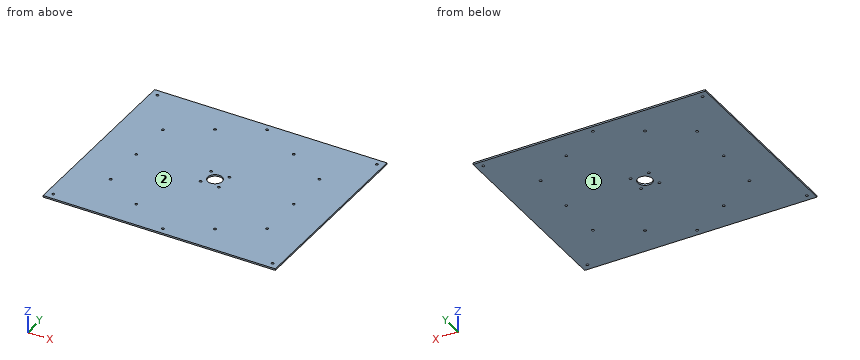
from build123d import *

# Parameters (mm, degrees)
F0_W     = 457.2
F0_H     = 381
F0_R     = 2.4892
F0_R_2   = 14.2875
F1_DEPTH = 3.175
F2_R     = 2.4892
F3_DEPTH = 3.176


with BuildPart() as f1:
    # F0 (on Top) → F1 (new body)
    with BuildSketch(Plane.XY):
        with Locations((228.6, 190.5)):
            Rectangle(F0_W, F0_H)
        with Locations((151.088372, 56.245922)):
            Circle(F0_R, mode=Mode.SUBTRACT)
        with Locations((74.620683, 101.6)):
            Circle(F0_R, mode=Mode.SUBTRACT)
        with Locations((210.639488, 172.539488)):
            Circle(F0_R, mode=Mode.SUBTRACT)
        with Locations((228.6, 12.7)):
            Circle(F0_R, mode=Mode.SUBTRACT)
        with Locations((306.111628, 56.245922)):
            Circle(F0_R, mode=Mode.SUBTRACT)
        with Locations((246.560512, 172.539488)):
            Circle(F0_R, mode=Mode.SUBTRACT)
        with Locations((382.579317, 101.6)):
            Circle(F0_R, mode=Mode.SUBTRACT)
        with Locations((73.576744, 190.5)):
            Circle(F0_R, mode=Mode.SUBTRACT)
        with Locations((74.620683, 279.4)):
            Circle(F0_R, mode=Mode.SUBTRACT)
        with Locations((210.639488, 208.460512)):
            Circle(F0_R, mode=Mode.SUBTRACT)
        with Locations((151.088372, 324.754078)):
            Circle(F0_R, mode=Mode.SUBTRACT)
        with Locations((228.6, 190.5)):
            Circle(F0_R_2, mode=Mode.SUBTRACT)
        with Locations((246.560512, 208.460512)):
            Circle(F0_R, mode=Mode.SUBTRACT)
        with Locations((383.623256, 190.5)):
            Circle(F0_R, mode=Mode.SUBTRACT)
        with Locations((382.579317, 279.4)):
            Circle(F0_R, mode=Mode.SUBTRACT)
        with Locations((306.111628, 324.754078)):
            Circle(F0_R, mode=Mode.SUBTRACT)
        with Locations((228.6, 368.3)):
            Circle(F0_R, mode=Mode.SUBTRACT)
    extrude(amount=F1_DEPTH)

    # F2 (on face) → F3 (cut, through all)
    with BuildSketch(Plane.XY.offset(3.175)):
        with Locations((12.7, 368.3)):
            Circle(F2_R)
        with Locations((444.5, 368.3)):
            Circle(F2_R)
        with Locations((444.5, 12.7)):
            Circle(F2_R)
        with Locations((12.7, 12.7)):
            Circle(F2_R)
    extrude(amount=-F3_DEPTH, mode=Mode.SUBTRACT)


solid = f1.part
Can you work these out from the model? Positions are in its coordinate system, mm. Face numbers are marked on the shaded views. Round coordinates to 2 decimals unless told otherwise and drop trailing zeros. Write each question's results on one line, items separated by ' | '. Start each with the question number.
1) Please list where these lines run through material, in increasing order: line 1 (Y direction, x = 444.5, z = 0.7); line 2 (X direction, y = 103.5, z = 2.65); line 3 (Y direction, x = 230.5, z = 2.5).
2) For pin 1 Ø4.5 at (x, y) = (382.58, 101.6) entering from -Z, with a flat end and sliding along its axis, tell me the tip position at first contact or that it passes through.
3) We'd pull the mould along Z, two halves only. Please class the marked faces 1 and 2: released by +Z, released by -Z, zero draft, split by the parting line, or undercut.
Here are the results:
1) line 1: y = 0 to 10.21, 15.19 to 365.81, 370.79 to 381 | line 2: x = 0 to 73.01, 76.23 to 380.97, 384.19 to 457.2 | line 3: y = 0 to 11.09, 14.31 to 176.34, 204.66 to 366.69, 369.91 to 381
2) pin 1: passes through
3) face 1: released by -Z | face 2: released by +Z
